from build123d import *

# Parameters (mm, degrees)
SKETCH1_W                = 70
SKETCH1_H                = 70
BOSS_EXTRUDE1_DEPTH      = 10
LPATTERN2_COUNT          = 2
LPATTERN2_PITCH          = 50
SKETCH2_R                = 15
SKETCH2_R_2              = 11
BOSS_EXTRUDE2_DEPTH      = 20
BOSS_EXTRUDE3_DEPTH      = 5
BOSS_EXTRUDE3_DEPTH_BACK = 55
SKETCH2_3_R              = 7.5
SKETCH2_3_R_2            = 5
CUT_EXTRUDE1_START       = -100
SKETCH3_R                = 5
SKETCH3_R_2              = 11
CUT_EXTRUDE1_DEPTH       = 100
FILLET1_R                = 10


with BuildPart() as part:
    # Sketch1 → Boss-Extrude1 (new body)
    with BuildSketch(Plane(origin=(0, 0, 0), x_dir=(1, 0, 0), z_dir=(0, 1, 0))):
        Rectangle(SKETCH1_W, SKETCH1_H)
    extrude(amount=BOSS_EXTRUDE1_DEPTH)


with BuildPart() as lpattern2_1:
    # LPattern2: pattern copy
    add(part.part.moved(Location(Vector(0, -1, 0) * (1 * LPATTERN2_PITCH))))


with BuildPart() as part_1:
    add(part.part)

    # Sketch2 → Boss-Extrude2 (add)
    with BuildSketch(Plane(origin=(0, 10, 0), x_dir=(1, 0, 0), z_dir=(0, 1, 0))):
        with Locations(Location((0, 0, 0), (0, 0, 90))):
            Circle(SKETCH2_R)
        with Locations(Location((0, 0, 0), (0, 0, 270))):
            Circle(SKETCH2_R_2, mode=Mode.SUBTRACT)
    extrude(amount=BOSS_EXTRUDE2_DEPTH)

    add(lpattern2_1.part)  # Boss-Extrude3 merges LPattern2_1
    # Sketch2_3 → Boss-Extrude3 (add, two sides: drawn at the far end of the back side and taken through both)
    # profile 1 of 4: a face of its own
    with BuildSketch(Plane(origin=(0, 10, 0), x_dir=(1, 0, 0), z_dir=(0, 1, 0)).offset(-BOSS_EXTRUDE3_DEPTH_BACK)):
        with Locations(Location((-25, 25, 0), (0, 0, 90))):
            Circle(SKETCH2_3_R)
        with Locations(Location((-25, 25, 0), (0, 0, 90))):
            Circle(SKETCH2_3_R_2, mode=Mode.SUBTRACT)
    # profile 2 of 4: a face of its own
    with BuildSketch(Plane(origin=(0, 10, 0), x_dir=(1, 0, 0), z_dir=(0, 1, 0)).offset(-BOSS_EXTRUDE3_DEPTH_BACK)):
        with Locations(Location((25, 25, 0), (0, 0, 90))):
            Circle(SKETCH2_3_R)
        with Locations(Location((25, 25, 0), (0, 0, 90))):
            Circle(SKETCH2_3_R_2, mode=Mode.SUBTRACT)
    # profile 3 of 4: a face of its own
    with BuildSketch(Plane(origin=(0, 10, 0), x_dir=(1, 0, 0), z_dir=(0, 1, 0)).offset(-BOSS_EXTRUDE3_DEPTH_BACK)):
        with Locations(Location((-25, -25, 0), (0, 0, 90))):
            Circle(SKETCH2_3_R)
        with Locations(Location((-25, -25, 0), (0, 0, 90))):
            Circle(SKETCH2_3_R_2, mode=Mode.SUBTRACT)
    # profile 4 of 4: a face of its own
    with BuildSketch(Plane(origin=(0, 10, 0), x_dir=(1, 0, 0), z_dir=(0, 1, 0)).offset(-BOSS_EXTRUDE3_DEPTH_BACK)):
        with Locations(Location((25, -25, 0), (0, 0, 90))):
            Circle(SKETCH2_3_R)
        with Locations(Location((25, -25, 0), (0, 0, 90))):
            Circle(SKETCH2_3_R_2, mode=Mode.SUBTRACT)
    extrude(amount=BOSS_EXTRUDE3_DEPTH + BOSS_EXTRUDE3_DEPTH_BACK)

    # Sketch3 → Cut-Extrude1 (cut)
    with BuildSketch(Plane(origin=(0, 10, 0), x_dir=(1, 0, 0), z_dir=(0, 1, 0)).offset(CUT_EXTRUDE1_START)):
        with Locations(Location((-25, -25, 0), (0, 0, 90))):
            Circle(SKETCH3_R)
        with Locations(Location((-25, 25, 0), (0, 0, 90))):
            Circle(SKETCH3_R)
        with Locations(Location((25, -25, 0), (0, 0, 90))):
            Circle(SKETCH3_R)
        with Locations(Location((25, 25, 0), (0, 0, 90))):
            Circle(SKETCH3_R)
        with Locations(Location((0, 0, 0), (0, 0, 90))):
            Circle(SKETCH3_R_2)
    extrude(amount=CUT_EXTRUDE1_DEPTH, mode=Mode.SUBTRACT)

    # Fillet1
    fillet1_edges = [part_1.edges().sort_by_distance(p)[0] for p in [
        (35, 5, 35),
        (35, 5, -35),
        (-35, 5, -35),
        (-35, 5, 35),
        (35, -45, 35),
        (-35, -45, 35),
        (-35, -45, -35),
        (35, -45, -35),
    ]]
    fillet(fillet1_edges, radius=FILLET1_R)


solid = part_1.part
Can you work these out from the model? Positions are in its coordinate system, mm. A direction names the side the tool comes from. Round coordinates to 2 decimals unless told otherwise and drop trailing zeros. Write each loop counter-clockwise with the first axis right and the second up, starting at its lowest first coordinate (ties: lowest second). Pieces come first, ordered by that corner, then holes. Notation, with made-up numbers: (89, 68.5) -> (107, 68.5) arc R14 cw to (107, 80.5) -> close; hole circle Ø3 at (74.5, 31). An arc over 180 degrees is marked (long way). Use one line per item in the form item = value. Start each with the question number.
Q1. Imagine slicing it at C-C (x = 27). Count the separate pieces of the cut face and the enclosed holes in it, then the cut area to 3 significant figures.
Q2. Imagine slicing it at D-D (y = -26.5). Please give me the cut outline in (x, z), then the cut area to 3 significant figures.
Q3. Imagine slicing it at A-A (x = 0). Please give me the cut outline in (y, z), then the cut area to 3 significant figures.
Q4. I'm going to push flat-ended pins straight in: P1, Ø4.5, axis at x = -23.5, z = 21.5, coming from the +Y side; P2, Ø1.5, axis at x = 24, y = -31.5, coming from the +Z side; P3, Ø10, axis at y = 15.5, z = -3.5, coming from the +X side; P4, Ø13, axis at x = 0, z = 0, coming from the +Y side. Where does each tip first touch, or does it pass through?
Q5. We'd pull the mould along Z, two halves only. Please class faces 1 (the face through (-31.99, -44.93, 32.15)), 2 (the face through (19.9, 12.5, 30.5)), 3 (the face through (-31.99, 5.07, -32.15)): +Z half, -Z half, draft (parallel to the pull), parting line (faces both ways), or undercut.
Q6. Imagine slicing it at B-B (y = 8.5). Please give me the cut outline in (x, z).
Q7. If I drill on probe 1 along X at (y, z) = (-22, -25); probe 2 along Y at (x, z) = (28, -8); probe 3 along X at (y, z) = (-23.5, -26), over which ranges is the centre line in solid material (lowest first)? Write a range as [from, to].
Q8. Which directions (+Z, -Z, +X, -X, +Y, -Y) give clear straight access to the entire face, cutting with the end or side of a thin tool? Please do faces 4 (the face through (-10, 30, 5)), 5 (the face through (-0.66, 19.86, 14.985)), 6 (the face through (-8, -40, -8)).
Worked out:
q1.separate_pieces = 3
q1.enclosed_holes = 1
q1.area = 1,500 mm^2
q2.outline = circle Ø15 at (-25, -25); circle Ø15 at (-25, 25); circle Ø15 at (25, -25); circle Ø15 at (25, 25); hole circle Ø10 at (-25, -25); hole circle Ø10 at (-25, 25); hole circle Ø10 at (25, -25); hole circle Ø10 at (25, 25)
q2.area = 393 mm^2
q3.outline = (-50, -35) -> (-40, -35) -> (-40, -11) -> (-50, -11) -> close; (-50, 11) -> (-40, 11) -> (-40, 35) -> (-50, 35) -> close; (0, -35) -> (10, -35) -> (10, -15) -> (30, -15) -> (30, -11) -> (0, -11) -> close; (0, 11) -> (30, 11) -> (30, 15) -> (10, 15) -> (10, 35) -> (0, 35) -> close
q3.area = 1,120 mm^2
q4.P1 = 15
q4.P2 = 32.5
q4.P3 = 15
q4.P4 = through
q5.face_1 = +Z half
q5.face_2 = undercut
q5.face_3 = -Z half
q6.outline = (-35, -25) arc R10 ccw to (-25, -35) -> (25, -35) arc R10 ccw to (35, -25) -> (35, 25) arc R10 ccw to (25, 35) -> (-25, 35) arc R10 ccw to (-35, 25) -> close; hole circle Ø10 at (-25, -25); hole circle Ø10 at (-25, 25); hole circle Ø22 at (0, 0); hole circle Ø10 at (25, -25); hole circle Ø10 at (25, 25)
q7.probe_1 = [-32.5, -30], [-20, -17.5], [17.5, 20], [30, 32.5]
q7.probe_2 = [-50, -40], [0, 10]
q7.probe_3 = [-32.43, -29.9], [-20.1, -17.57], [17.57, 20.1], [29.9, 32.43]
q8.face_4 = +Z, -Z, +X, -X, +Y
q8.face_5 = +Y
q8.face_6 = none
